Verification items for the finished model (mm, model axes). Give positions to 0.01 mm unless a question says otherwise; leave off trailing zeros. Write each loop counter-clockwise with the first axis right and the second up, starting at its lowest first coordinate (ties: lowest second). Pieces come first, ordered by that corner, then holes. Notation, with made-up numbers: (85.5, 48.5) -> (96.5, 48.5) arc R16 ccw to (96.5, 59.5) -> close; hole circle Ø7 at (63.25, 13). An arc over 180 degrees is marked (long way). Write item = value, one per line.
from build123d import *

# Parameters (mm, degrees)
BOSS_EXTRUDE1_DEPTH = 3
FILLET1_R           = 5
CUT_EXTRUDE1_REACH  = 156.417
SKETCH2_R           = 1.5


with BuildPart() as part:
    # Sketch1 → Boss-Extrude1 (new body)
    with BuildSketch(Plane(origin=(0, 0, 0), x_dir=(1, 0, 0), z_dir=(0, 1, 0))):
        with BuildLine():
            Line((-68.408481347, 122.148596717), (-57.801879629, 111.541994999))
            ThreePointArc((-57.801879629, 111.541994999), (0, 129.939649987), (57.801879629, 111.541994999))
            Line((57.801879629, 111.541994999), (68.408481347, 122.148596717))
            ThreePointArc((68.408481347, 122.148596717), (0, 140), (-68.408481347, 122.148596717))
        make_face()
    extrude(amount=BOSS_EXTRUDE1_DEPTH)

    # Fillet1
    fillet1_edges = [part.edges().sort_by_distance(p)[0] for p in [
        (68.408481347, 1.5, -122.148596717),
        (57.801879629, 1.5, -111.541994999),
        (-57.801879629, 1.5, -111.541994999),
        (-68.408481347, 1.5, -122.148596717),
    ]]
    fillet(fillet1_edges, radius=FILLET1_R)

    # Sketch2 → Cut-Extrude1 (cut, up to next)
    with BuildSketch(Plane(origin=(0, 3, 0), x_dir=(1, 0, 0), z_dir=(0, 1, 0)), mode=Mode.PRIVATE) as cut_extrude1_sk1:
        with Locations(Location((-50, 124, 0), (0, 0, 270))):
            Circle(SKETCH2_R)
    cut_extrude1_tool1 = extrude(cut_extrude1_sk1.sketch, amount=-CUT_EXTRUDE1_REACH, mode=Mode.PRIVATE) & part.part
    # Sketch2 → Cut-Extrude1 (cut, up to next)
    with BuildSketch(Plane(origin=(0, 3, 0), x_dir=(1, 0, 0), z_dir=(0, 1, 0)), mode=Mode.PRIVATE) as cut_extrude1_sk2:
        with Locations(Location((50, 124, 0), (0, 0, 270))):
            Circle(SKETCH2_R)
    cut_extrude1_tool2 = extrude(cut_extrude1_sk2.sketch, amount=-CUT_EXTRUDE1_REACH, mode=Mode.PRIVATE) & part.part
    add(cut_extrude1_tool1.solids().sort_by_distance((-50, 3, -124))[0], mode=Mode.SUBTRACT)
    add(cut_extrude1_tool2.solids().sort_by_distance((50, 3, -124))[0], mode=Mode.SUBTRACT)


solid = part.part
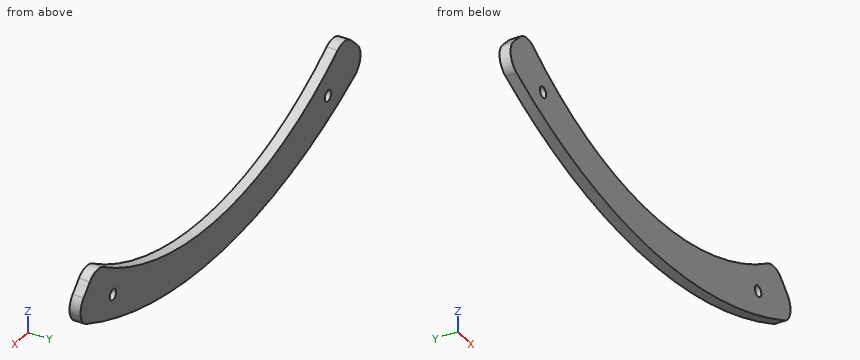
Item 1: Material ranges on line 1 (X direction, y = 2.4, z = -114.75); line 2 (X direction, y = 1.8, z = -114.5); line 3 (Z direction, x = 6, y = 1.85), recorded low to high.
Response values:
line_1 = -61.01 to -52.98, 52.98 to 61.01
line_2 = -60.76 to -53.38, 53.38 to 60.76
line_3 = -139.87 to -129.76
Item 2: Sectioned sample at B-B on x = -50. Record the cut outline in (y, z).
Response values:
outline = (0, -130.77) -> (3, -130.77) -> (3, -125.5) -> (0, -125.5) -> close; (0, -122.5) -> (3, -122.5) -> (3, -116.54) -> (0, -116.54) -> close
Item 3: Sectioned sample at C-C on z = -124. Record the cut outline in (x, y).
Response values:
outline = (-64, 0) -> (-51.5, 0) -> (-51.5, 3) -> (-64, 3) -> close; (-48.5, 0) -> (-33.95, 0) -> (-33.95, 3) -> (-48.5, 3) -> close; (33.95, 0) -> (48.5, 0) -> (48.5, 3) -> (33.95, 3) -> close; (51.5, 0) -> (64, 0) -> (64, 3) -> (51.5, 3) -> close
Item 4: Sectioned sample at A-A on y = 0.8. Record the cut outline in (x, z).
Response values:
outline = (-63.62, -117.36) arc R5 ccw to (-62.31, -125.37) arc R140 ccw to (62.31, -125.37) arc R5 ccw to (63.62, -117.36) -> (60.72, -114.46) arc R5 ccw to (54.46, -113.81) arc R100 cw to (-54.46, -113.81) arc R5 ccw to (-60.72, -114.46) -> close; hole circle Ø3 at (-50, -124); hole circle Ø3 at (50, -124)
Item 5: Go/stop test with a flat-tipped pin: P1, Ø1, axis at x = 9, y = 2.5, coming from the +Z side. Record where the tip stops, or that it passes through.
Response values:
P1 = -129.49
Item 6: Sectioned sample at D-D on z = -116. Record the cut outline in (x, y), then the cut area to 3 significant figures.
Response values:
outline = (-62.26, 0) -> (-50.93, 0) -> (-50.93, 3) -> (-62.26, 3) -> close; (50.93, 0) -> (62.26, 0) -> (62.26, 3) -> (50.93, 3) -> close
area = 68.0 mm^2
